Autodesk Inventor part; units mm, degrees
ref_plane "Plano de trabalho1" through (0, 0, 0) normal (0, 1, 0) x (1, 0, 0)
ref_plane "YZ Plane" through (0, 0, 0) normal (1, 0, 0) x (0, 1, 0)
ref_plane "XZ Plane" through (0, 0, 0) normal (0, 1, 0) x (-1, 0, 0)
sketch "Esboço1" plane through (0, 0, 0) normal (0, 1, 0) x (-1, 0, 0)
  line L0 (50.5, 44) -> (-50.5, 44)
  line L1 (-50.5, 44) -> (-50.5, -44)
  line L2 (-50.5, -44) -> (50.5, -44)
  line L3 (50.5, -44) -> (50.5, 44)
  line L4 (50.5, 44) -> (-50.5, -44) construction
  line L5 (-50.5, 44) -> (50.5, -44) construction
  line L6 (-29.5, 38) -> (-50.5, 38)
  line L7 (-50.5, 38) -> (-50.5, -38)
  line L8 (-50.5, -38) -> (-29.5, -38)
  line L9 (-29.5, -38) -> (-29.5, 38)
  line L10 (-29.5, 38) -> (-50.5, -38) construction
  line L11 (-50.5, 38) -> (-29.5, -38) construction
  line L12 (48.5, -44) -> (48.5, 44)
  point P0 (0, 0)
  point P1 (-40, 0)
  dimension "d0" = 101
  dimension "d1" = 88
  dimension "d2" = 21
  dimension "d3" = 76
  dimension "d4" = 2
extrude "Extrusão1" add sketch "Esboço1" along normal blind 2
extrude "Extrusão2" add sketch "Esboço1" against normal blind 23 contours L3 L2 L12 L0
extrude "Extrusão3" add sketch "Esboço1" against normal blind 17 contours L6 L9 L8 L1
ref_plane "Plano de trabalho1" through (0, 0, 0) normal (0, 1, 0) x (1, 0, 0)
split_face "Dividir1"
sketch "Esboço2" plane through (0, 2, 0) normal (0, 1, 0) x (1, 0, 0)
  line L0 (-50.5, 44) -> (-50.5, -44)
  line L1 (-40, -40) -> (-40, 40) construction
  line L2 (-40, 40) -> (40, 40) construction
  line L3 (40, 40) -> (40, -40) construction
  line L4 (40, -40) -> (-40, -40) construction
  line L5 (-40, -40) -> (40, 40) construction
  point P0 (0, 0)
  point P1 (0, 0)
  dimension "d25" = 80
properties part number "Bitdoglab"
Could you check a few things on this model? Use its own coordinates, in mm. A direction names the side the tool comes from. Give positions to 0.01 mm unless a question says otherwise; leave off trailing zeros. Order: outer loops, then holes, each group sorted by start corner. A loop starts at its lowest first (then second) coordinate and runs counter-clockwise, first axis right, second up.
Item 1: If we section it at B-B, the plane z = -19: Write out the boundary of the cut face in (x, y).
Item 2: If we section it at A-A, the plane y = -8.75: Write out the boundary of the cut face in (x, z), plus the area to 3 significant figures.
Item 3: I'm going to push flat-ended pins straight in: pin 1 (10 mm diameter, centred on x = -12, z = 17, fed in from -Y); pin 2 (17 mm diameter, centred on x = 36.5, z = 3.5, fed in from -Y); pin 3 (8.5 mm diameter, centred on x = 38, y = -5.5, fed in from -Z). Where does each tip first touch, or does it pass through?
Item 4: If we section it at D-D, the plane y = -18.75: Write out the boundary of the cut face in (x, z).
Item 5: I need wall thicknesses on line 1 (X direction, y = -8.25, z = 10); line 2 (Y direction, x = -10.5, z = 1); line 3 (X direction, y = -16.5, z = -39.5). Which ranges of each line are inside material? Lowest first, please.
Item 6: If we section it at C-C, the plane x = -12: Write out the boundary of the cut face in (y, z), plus the area to 3 significant figures.
Item 7: If we mould it in two halves opening along X, with no side actions, what happens to faces 4 (the face through (29.5, -8, -1)), 5 (the face through (50.5, -8, 1)), 6 (the face through (40, -8, -38))? For each: pulls with the +X half, pulls with the -X half, needs draft (parallel to the pull), parting line crosses it, or undercut.
Item 8: For faces 1 (the face through (-48.5, -11, -1)), 2 (the face through (40, -17, 1)), 3 (the face through (40, -8, 38)), which set-ups out of +Z, -Z, +X, -X, +Y, -Y let a thin tool reach every point of the face, with its end or its side?
Values:
1. outline: (-50.5, -23) - (-48.5, -23) - (-48.5, 0) - (29.5, 0) - (29.5, -17) - (50.5, -17) - (50.5, 2) - (-50.5, 2) - close
2. outline: (-50.5, -44) - (-48.5, -44) - (-48.5, 44) - (-50.5, 44) - close; (29.5, -38) - (50.5, -38) - (50.5, 38) - (29.5, 38) - close
2. area: 1,770 mm2
3. pin 1: stops at y = 0
3. pin 2: stops at y = -17
3. pin 3: stops at z = -38
4. outline: (-50.5, -44) - (-48.5, -44) - (-48.5, 44) - (-50.5, 44) - close
5. line 1: x = -50.5 to -48.5, 29.5 to 50.5
5. line 2: y = 0 to 2
5. line 3: x = -50.5 to -48.5
6. outline: (0, -44) - (2, -44) - (2, 44) - (0, 44) - close
6. area: 176 mm2
7. face 4: undercut
7. face 5: pulls with the +X half
7. face 6: needs draft
8. face 1: +Z, -Z, -Y
8. face 2: +Z, -Z, +X, -Y
8. face 3: +Z, +X, -Y
